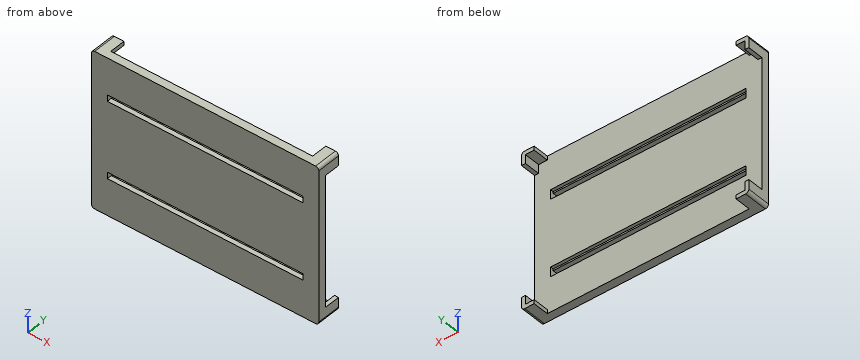
from build123d import *

# Parameters (mm, degrees)
BOSS_EXTRUDE1_DEPTH = 15
SKETCH2_W           = 138
SKETCH2_H           = 93.2
CUT_EXTRUDE1_DEPTH  = 10
SKETCH3_W           = 2.5
SKETCH3_H           = 82.2
SKETCH3_W_2         = 127
SKETCH3_H_2         = 2.5
CUT_EXTRUDE2_DEPTH  = 10
SKETCH7_W           = 123
SKETCH7_H           = 6
CUT_EXTRUDE6_DEPTH  = 2
SKETCH8_W           = 123
SKETCH8_H           = 4
CUT_EXTRUDE7_DEPTH  = 3


with BuildPart() as part:
    # Sketch1 → Boss-Extrude1 (new body)
    with BuildSketch(Plane(origin=(0, 0, 0), x_dir=(1, 0, 0), z_dir=(0, 1, 0))):
        with BuildLine():
            Line((-69.5, -49.1), (69.5, -49.1))
            ThreePointArc((69.5, -49.1), (70.914213562, -48.514213562), (71.5, -47.1))
            Line((71.5, -47.1), (71.5, 47.1))
            ThreePointArc((71.5, 47.1), (70.914213562, 48.514213562), (69.5, 49.1))
            Line((69.5, 49.1), (-69.5, 49.1))
            ThreePointArc((-69.5, 49.1), (-70.914213562, 48.514213562), (-71.5, 47.1))
            Line((-71.5, 47.1), (-71.5, -47.1))
            ThreePointArc((-71.5, -47.1), (-70.914213562, -48.514213562), (-69.5, -49.1))
        make_face()
    extrude(amount=BOSS_EXTRUDE1_DEPTH)

    # Sketch2 → Cut-Extrude1 (cut)
    with BuildSketch(Plane(origin=(0, 15, 0), x_dir=(1, 0, 0), z_dir=(0, 1, 0))):
        Rectangle(SKETCH2_W, SKETCH2_H)
    extrude(amount=-CUT_EXTRUDE1_DEPTH, mode=Mode.SUBTRACT)

    # Sketch3 → Cut-Extrude2 (cut)
    with BuildSketch(Plane(origin=(0, 15, 0), x_dir=(1, 0, 0), z_dir=(0, 1, 0))):
        with Locations((-70.25, 0)):
            Rectangle(SKETCH3_W, SKETCH3_H)
        with Locations((0, 47.85)):
            Rectangle(SKETCH3_W_2, SKETCH3_H_2)
        with Locations((70.25, 0)):
            Rectangle(SKETCH3_W, SKETCH3_H)
        with Locations((0, -47.85)):
            Rectangle(SKETCH3_W_2, SKETCH3_H_2)
    extrude(amount=-CUT_EXTRUDE2_DEPTH, mode=Mode.SUBTRACT)

    # Sketch7 → Cut-Extrude6 (cut)
    with BuildSketch(Plane(origin=(0, 5, 0), x_dir=(1, 0, 0), z_dir=(0, 1, 0))):
        with Locations((0, 24.1)):
            Rectangle(SKETCH7_W, SKETCH7_H)
        with Locations((0, -24.1)):
            Rectangle(SKETCH7_W, SKETCH7_H)
    extrude(amount=-CUT_EXTRUDE6_DEPTH, mode=Mode.SUBTRACT)

    # Sketch8 → Cut-Extrude7 (cut)
    with BuildSketch(Plane(origin=(0, 3, 0), x_dir=(1, 0, 0), z_dir=(0, 1, 0))):
        with Locations((0, 24.1)):
            Rectangle(SKETCH8_W, SKETCH8_H)
        with Locations((0, -24.1)):
            Rectangle(SKETCH8_W, SKETCH8_H)
    extrude(amount=-CUT_EXTRUDE7_DEPTH, mode=Mode.SUBTRACT)


solid = part.part
Part model, mm, in its own coordinate system. Coordinates: 2 decimals unless noted, no trailing zeros. Loops run counter-clockwise (first coordinate to the right, second up) from the corner with the lowest first, then second, coordinate; pieces in that order, holes last. Notation, with made-up numbers: M 23.25,89.5 L 45.25,89.5 A33 cw 45.25,121.5 Z; hole C 75,-29 d3. An arc over 180 degrees is marked long. Use a Markdown table: item, result. Add a question column.
Q1. Cut at C-C (y = 11.25). Write the cut outline in (x, z).
Q2. Cut at D-D (z = -12). Write the cut outline in (x, y).
Q3. Cut at A-A (y = 1.5). Write the cut outline in (x, z), and give its area (3 significant figures).
Q4. Cut at B-B (x = 43). Write the cut outline in (y, z).
Q5. Probe L1, parallel to Z at x = -47, y = 4.5; L2, parallel to Y at x = -37.5, z = -4; L3, parallel to Y at x = -50, z = -27. List the from-to ranges inside material, lowest first.
Q6. Pin check, flat tips, straight feed: P1, Ø12, axis at x = -23, z = 4.5, coming from the +Y side; P2, Ø1.2, axis at x = 70.5, y = 11, coming from the -Z side; P3, Ø0.8, axis at x = 70.5, y = 7.5, coming from the +Z side. Stop position of each tip, or through.
Worked out:
| question | item | result |
|---|---|---|
| 1 | outline | M -71.5,-47.1 A2 ccw -69.5,-49.1 L -63.5,-49.1 L -63.5,-46.6 L -69,-46.6 L -69,-41.1 L -71.5,-41.1 Z; M -71.5,41.1 L -69,41.1 L -69,46.6 L -63.5,46.6 L -63.5,49.1 L -69.5,49.1 A2 ccw -71.5,47.1 Z; M 63.5,-49.1 L 69.5,-49.1 A2 ccw 71.5,-47.1 L 71.5,-41.1 L 69,-41.1 L 69,-46.6 L 63.5,-46.6 Z; M 63.5,46.6 L 69,46.6 L 69,41.1 L 71.5,41.1 L 71.5,47.1 A2 ccw 69.5,49.1 L 63.5,49.1 Z |
| 2 | outline | M -71.5,0 L 71.5,0 L 71.5,5 L -71.5,5 Z |
| 3 | outline | M -71.5,-47.1 A2 ccw -69.5,-49.1 L 69.5,-49.1 A2 ccw 71.5,-47.1 L 71.5,47.1 A2 ccw 69.5,49.1 L -69.5,49.1 A2 ccw -71.5,47.1 Z; hole M -61.5,-26.1 L 61.5,-26.1 L 61.5,-22.1 L -61.5,-22.1 Z; hole M -61.5,22.1 L 61.5,22.1 L 61.5,26.1 L -61.5,26.1 Z |
| 3 | area | 13,100 mm2 |
| 4 | outline | M 0,-49.1 L 5,-49.1 L 5,-27.1 L 3,-27.1 L 3,-26.1 L 0,-26.1 Z; M 0,-22.1 L 3,-22.1 L 3,-21.1 L 5,-21.1 L 5,21.1 L 3,21.1 L 3,22.1 L 0,22.1 Z; M 0,26.1 L 3,26.1 L 3,27.1 L 5,27.1 L 5,49.1 L 0,49.1 Z |
| 5 | L1 | z = -49.1 to -27.1, -21.1 to 21.1, 27.1 to 49.1 |
| 5 | L2 | y = 0 to 5 |
| 5 | L3 | y = 0 to 3 |
| 6 | P1 | stops at y = 5 |
| 6 | P2 | stops at z = -49.06 |
| 6 | P3 | stops at z = 49.01 |
